Verification items for the finished model (mm, model axes). Coordinates: 2 decimals unless noted, no trailing zeros. Order: outer loops, then holes, each group sorted by start corner. A loop starts at its lowest first (then second) coordinate and runs counter-clockwise, first axis right, second up. Notation, with made-up numbers: (-27.75, 64) -> (11.25, 64) arc R13 ccw to (11.25, 85) -> close; hole circle Ø4 at (13, -6.5). An arc over 180 degrees is marked (long way). Write item = value, one per line. Start each with the question number.
1. Cross-section at B-B on x = 12.5. Record the cut outline in (y, z), plus the area to 3 significant figures.
2. Cross-section at D-D on x = 2. Record the cut outline in (y, z), plus the area to 3 significant figures.
3. Cross-section at A-A on z = -7. Record the cut outline in (x, y), plus the area to 3 significant figures.
4. Go/stop test with a flat-tipped pin: P1, Ø4, axis at y = 24.5, z = -8.5, coming from the -X side. Record where the tip stops, or that it passes through.
5. Thickness scan on line 1 along Y through (x, z) = (20.5, 20.5); line 2 along Z through (x, y) = (13.25, -25); line 3 along Y through (x, z) = (22.25, -7.5). Record the ranges inside material, lowest first. Write a range as from..to.
6. Cross-section at C-C on y = 24. Record the cut outline in (x, z).
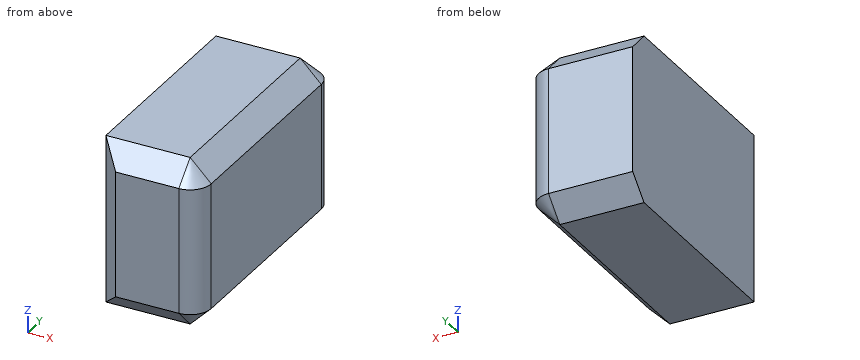
from build123d import *

# Parameters (mm, degrees)
F0_W     = 59.488162
F0_H     = 40.484803
F1_DEPTH = 25.4
F2_R     = 5.08
F3_SIZE  = 5.08


with BuildPart() as f1:
    # F0 (on Right) → F1 (new body)
    with BuildSketch(Plane.YZ):
        with Locations((2.245061, 2.255453)):
            Rectangle(F0_W, F0_H)
    extrude(amount=F1_DEPTH)

    # F2
    f2_edges = [f1.edges().sort_by_distance(p)[0] for p in [
        (25.4, -27.49902, 2.255454),
        (25.4, 31.989142, 2.255454),
    ]]
    fillet(f2_edges, radius=F2_R)

    # F3
    f3_edges = [f1.edges().sort_by_distance(p)[0] for p in [
        (10.16, -27.49902, 22.497855),
        (20.32, -27.49902, 2.255454),
        (0, -27.49902, 2.255454),
        (10.16, -27.49902, -17.986948),
    ]]
    chamfer(f3_edges, length=F3_SIZE)


solid = f1.part
Worked out:
q1.outline = (-27.5, -12.91) -> (-22.42, -17.99) -> (26.91, -17.99) -> (31.99, -12.91) -> (31.99, 17.42) -> (26.91, 22.5) -> (-22.42, 22.5) -> (-27.5, 17.42) -> close
q1.area = 2,360 mm²
q2.outline = (-24.42, -15.99) -> (-22.42, -17.99) -> (26.91, -17.99) -> (31.99, -12.91) -> (31.99, 17.42) -> (26.91, 22.5) -> (-22.42, 22.5) -> (-24.42, 20.5) -> close
q2.area = 2,250 mm²
q3.outline = (0, -22.42) -> (5.08, -27.5) -> (20.32, -27.5) arc R5.08 ccw to (25.4, -22.42) -> (25.4, 26.91) arc R5.08 ccw to (20.32, 31.99) -> (0, 31.99) -> close
q3.area = 1,490 mm²
q4.P1 = 0
q5.line_1 = -24.41..28.9
q5.line_2 = -15.41..19.92
q5.line_3 = -27.12..31.61
q6.outline = (0, -17.99) -> (20.32, -17.99) -> (25.4, -12.91) -> (25.4, 17.42) -> (20.32, 22.5) -> (0, 22.5) -> close
